Autodesk Inventor part; units mm, degrees
ref_plane "to_bolt_XY" through (-3.5679, 0, -0.0524) normal (0.7071, 0, 0.7071) x (-0.7071, 0, 0.7071)
ref_plane "to_bolt_YZ" through (-3.5679, 0, -0.0524) normal (-0.7071, 0, 0.7071) x (0, -1, 0)
ref_plane "to_bolt_ZX" through (-3.5679, 0, -0.0524) normal (0, -1, 0) x (0.7071, 0, 0.7071)
sketch "Sketch_1" plane through (0, 0, 0) normal (0, 1, 0) x (-1, 0, 0)
  line L0 (9.1622, -0.2102) -> (8.4597, 7.1326)
  line L1 (8.4597, 7.1326) -> (8.2577, 7.6457)
  arc A0 (8.2577, 7.6457) -> (7.905, 7.6831) centre (8.0716, 7.5725) ccw
  line L2 (7.905, 7.6831) -> (5.2627, 3.7047)
  arc A1 (5.1192, 3.6167) -> (5.2627, 3.7047) centre (5.0961, 3.8154) ccw
  line L3 (5.1192, 3.6167) -> (-0.3472, 2.9798)
  arc A2 (-0.3472, 2.9798) -> (0.287, -2.9862) centre (0, 0) ccw
  arc A3 (0.8188, -3.3585) -> (0.287, -2.9862) centre (0.3348, -3.4839) ccw
  line L4 (0.8188, -3.3585) -> (1.8215, -7.2275)
  arc A4 (1.8215, -7.2275) -> (2.1565, -7.3187) centre (2.0151, -7.1773) ccw
  line L5 (2.1565, -7.3187) -> (9.1045, -0.3707)
  arc A5 (9.1045, -0.3707) -> (9.1513, -0.2969) centre (8.9631, -0.2293) ccw
  arc A6 (9.1513, -0.2969) -> (9.1622, -0.2102) centre (8.9631, -0.2293) ccw
  circle A7 centre (0, 0) radius 1.555
extrude "Extrusion1" add sketch "Sketch_1" along normal mid plane 35
sketch "Sketch_2" plane through (0, 0, 0) normal (0, 1, 0) x (-1, 0, 0)
  line L0 (6.2296, 2.6092) -> (5.9185, 2.9204)
  line L1 (5.9185, 2.9204) -> (5.7646, 4.4605)
  line L2 (5.7646, 4.4605) -> (5.2627, 3.7047)
  line L3 (5.2627, 3.7047) -> (5.1192, 3.6167)
  line L4 (5.1192, 3.6167) -> (-0.3472, 2.9798)
  arc A0 (-0.3472, 2.9798) -> (0.287, -2.9862) centre (0, 0) ccw
  arc A1 (0.8188, -3.3585) -> (0.287, -2.9862) centre (0.3348, -3.4839) ccw
  line L5 (0.8188, -3.3585) -> (0.7763, -2.9407)
  arc A2 (0.9064, -2.714) -> (0.7763, -2.9407) centre (1.26, -3.0675) ccw
  line L6 (0.9064, -2.714) -> (6.2296, 2.6092)
extrude "Extrusion2" cut sketch "Sketch_2" along normal mid plane 22.1
sketch "Sketch_3" plane through (-0.9064, -11.05, -2.714) normal (0.7071, 0, 0.7071) x (-0.7071, 0, 0.7071)
  line L0 (0.334, -13.0303) -> (3.764, -15.0106)
  line L1 (3.764, -15.0106) -> (7.194, -13.0303)
  line L2 (7.194, -13.0303) -> (7.194, -9.0697)
  line L3 (7.194, -9.0697) -> (3.764, -7.0894)
  line L4 (3.764, -7.0894) -> (0.334, -9.0697)
  line L5 (0.334, -9.0697) -> (0.334, -13.0303)
extrude "Extrusion3" add sketch "Sketch_3" along normal mid plane 0.6
sketch "Sketch_4" plane through (0, 0, 0) normal (1, 0, 0) x (0, 1, 0)
  line L0 (-17.5, 0) -> (17.5, 0)
  line L1 (17.5, 0) -> (17.5, -0.72)
  line L2 (17.5, -0.72) -> (16.75, -1.555)
  line L3 (16.75, -1.555) -> (-16.75, -1.555)
  line L4 (-16.75, -1.555) -> (-17.5, -0.72)
  line L5 (-17.5, -0.72) -> (-17.5, 0)
  line L6 (-17.5, 0) -> (17.5, 0)
revolve "Revolution1" add sketch "Sketch_4" angle 360 about axis through (0, -17.5, 0) along (0, -1, 0)
sketch "Sketch5" plane through (-6.2296, -11.05, 2.6092) normal (0.7071, 0, 0.7071) x (0.7071, 0, -0.7071)
  point P0 (3.7632, 3.55)
hole "Hole1" at (-3.5687, -7.5, -0.0517) direction (-0.7071, 0, -0.7071) diameter 4.21 depth 0.2
sketch "Sketch6" plane through (-6.2296, -11.05, 2.6092) normal (0.7071, 0, 0.7071) x (0.7071, 0, -0.7071)
  point P0 (3.7632, 18.55)
hole "Hole2" at (-3.5687, 7.5, -0.0517) direction (-0.7071, 0, -0.7071) diameter 4.21 depth 0.2
ref_plane "to_bolt_XY" through (-3.5679, 0, -0.0524) normal (0.7071, 0, 0.7071) x (-0.7071, 0, 0.7071)
ref_plane "to_bolt_YZ" through (-3.5679, 0, -0.0524) normal (-0.7071, 0, 0.7071) x (0, -1, 0)
ref_plane "to_bolt_ZX" through (-3.5679, 0, -0.0524) normal (0, -1, 0) x (0.7071, 0, 0.7071)
ref_plane "to_door_XY" through (0, 0, 0) normal (0, 1, 0) x (1, 0, 0)
ref_plane "to_door_YZ" through (0, 0, 0) normal (1, 0, 0) x (0, 0, -1)
ref_plane "to_door_ZX" through (0, 0, 0) normal (0, 0, -1) x (0, 1, 0)
ref_plane "to_frame_XY" through (-5.6305, 0, -3.8447) normal (0.7071, 0, 0.7071) x (0.7071, 0, -0.7071)
ref_plane "to_frame_YZ" through (-5.6305, 0, -3.8447) normal (0.7071, 0, -0.7071) x (0, 1, 0)
ref_plane "to_frame_ZX" through (-5.6305, 0, -3.8447) normal (0, 1, 0) x (0.7071, 0, 0.7071)
properties part number "JB_HINGE"
Could you check a few things on this model? Use its own coordinates, in mm. A direction names the side the tool comes from. Give positions to 0.01 mm unless a question says otherwise; leave off trailing zeros. Loops run counter-clockwise (first coordinate to the right, second up) from the corner with the lowest first, then second, coordinate; pieces in that order, holes last. Notation, with made-up numbers: (12.25, -22) -> (66.25, -22) arc R21 ccw to (66.25, 3) -> close; hole circle Ø4 at (41.25, -32.5). An arc over 180 degrees is marked (long way). Answer as CSV lines item,"result". Start each with the question number.
(1) We'd pull the mould along X, two halves only. Please class faces 3 (the flat face through (-2, -11.05, 1)), 4 (the flat face through (-2.4, 14.2, 3.3)), 5 (the flat face through (-4, 17.5, 0)), 6 (the cylindrical face through (0.337, -17.13, 1.518)): released by +X, released by -X, zero draft, split by the parting line, or undercut.
(2) Which directions (+Z, -Z, +X, -X, +Y, -Y) give clear straight access to the entire face, cutting with the end or side of a thin tool? Please do faces 1 (the flat face through (-2, 11.05, 1)), 2 (the flat face through (-8.816, -0.245, 3.41)).
(3) I need wall thicknesses on probe 1 along X at (y, z) = (17.15, 0) (3 decimals); probe 2 along X at (y, z) = (17, 0) (3 decimals); probe 3 along Y at (x, z) = (-3.5, 1.5). Which ranges of each line are inside material? Lowest first, please.
(4) If we section it at D-D on x = -6.75: Write out the boundary of the cut face in (y, z), then the cut area to 3 significant figures.
(5) I'm going to push flat-ended pins straight in: pin 1 Ø6 at (x, y) = (-4.5, -2) entering from +Z; pin 2 Ø2 at (y, z) = (-0.5, 5.5) entering from -X; pin 3 Ø1.5 at (y, z) = (-4.5, 6) entering from -X. Where does each tip first touch, or does it pass through?
(6) If we section it at B-B on z = 2: Write out the boundary of the cut face in (x, y), then the cut area to 3 significant figures.
Computed:
1,face 3,"undercut"
1,face 4,"released by +X"
1,face 5,"zero draft"
1,face 6,"undercut"
2,face 1,"none"
2,face 2,"+Z, -X, +Y, -Y"
3,probe 1,"x = -9.142 to -1.555, -1.11 to 1.11, 1.555 to 3"
3,probe 2,"x = -9.142 to -1.555, -1.277 to 1.277, 1.555 to 3"
3,probe 3,"y = -17.5 to -11.05, 11.05 to 17.5"
4,outline,"(-17.5, -2.73) -> (17.5, -2.73) -> (17.5, 5.94) -> (-17.5, 5.94) -> close"
4,area,"303 mm2"
5,pin 1,"stops at z = 7.07"
5,pin 2,"stops at x = -8.71"
5,pin 3,"stops at x = -8.64"
6,outline,"(-8.95, -17.5) -> (2.24, -17.5) -> (2.24, -11.05) -> (-5.62, -11.05) -> (-5.62, -2.28) -> (-5.2, -2.46) -> (-5.2, 2.46) -> (-5.62, 2.28) -> (-5.62, 11.05) -> (2.24, 11.05) -> (2.24, 17.5) -> (-8.95, 17.5) -> close"
6,area,"220 mm2"
